from build123d import *

# Parameters (mm, degrees)
SKETCH1_R           = 1.75
SKETCH1_R_2         = 1.8
SKETCH1_R_3         = 1.7
BOSS_EXTRUDE1_DEPTH = 3


with BuildPart() as part:
    # Sketch1 → Boss-Extrude1 (new body)
    with BuildSketch(Plane.XY):
        with BuildLine():
            Line((-138, 334), (-123.000000001, 334))
            ThreePointArc((-123.000000001, 334), (-121.585786438, 333.414213562), (-121.000000001, 332))
            Line((-121.000000001, 332), (-121.000000001, 330))
            ThreePointArc((-121.000000001, 330), (-120.414213563, 328.585786438), (-119.000000001, 328))
            Line((-119.000000001, 328), (-79.825853915, 328))
            ThreePointArc((-79.825853915, 328), (-78.411640352, 327.414213562), (-77.825853915, 326))
            Line((-77.825853915, 326), (-77.825853915, 319))
            ThreePointArc((-77.825853915, 319), (-70.325853915, 311.5), (-62.825853915, 319))
            Line((-62.825853915, 319), (-62.825853915, 326))
            ThreePointArc((-62.825853915, 326), (-62.240067477, 327.414213562), (-60.825853915, 328))
            Line((-60.825853915, 328), (69.799384712, 328))
            ThreePointArc((69.799384712, 328), (71.213598275, 327.414213562), (71.799384712, 326))
            Line((71.799384712, 326), (71.799384712, 319))
            ThreePointArc((71.799384712, 319), (79.299384712, 311.5), (86.799384712, 319))
            Line((86.799384712, 319), (86.799384712, 326))
            ThreePointArc((86.799384712, 326), (87.38517115, 327.414213562), (88.799384712, 328))
            Line((88.799384712, 328), (119.000000001, 328))
            ThreePointArc((119.000000001, 328), (120.414213563, 328.585786438), (121.000000001, 330))
            Line((121.000000001, 330), (121.000000001, 332))
            ThreePointArc((121.000000001, 332), (121.585786438, 333.414213562), (123.000000001, 334))
            Line((123.000000001, 334), (138, 334))
            ThreePointArc((138, 334), (140.121320344, 333.121320344), (141, 331))
            Line((141, 331), (141, 227))
            ThreePointArc((141, 227), (140.121320344, 224.878679656), (138, 224))
            Line((138, 224), (-138, 224))
            ThreePointArc((-138, 224), (-140.121320344, 224.878679656), (-141, 227))
            Line((-141, 227), (-141, 331))
            ThreePointArc((-141, 331), (-140.121320344, 333.121320344), (-138, 334))
        make_face()
        with Locations((-131, 319)):
            Circle(SKETCH1_R, mode=Mode.SUBTRACT)
        with Locations((-131, 239)):
            Circle(SKETCH1_R, mode=Mode.SUBTRACT)
        with Locations((131, 319)):
            Circle(SKETCH1_R, mode=Mode.SUBTRACT)
        with Locations((131, 239)):
            Circle(SKETCH1_R, mode=Mode.SUBTRACT)
        with Locations((-104.5, 311.05)):
            Circle(SKETCH1_R, mode=Mode.SUBTRACT)
        with Locations((-94, 311.05)):
            Circle(SKETCH1_R, mode=Mode.SUBTRACT)
        with Locations((-103.8, 298.65)):
            Circle(SKETCH1_R, mode=Mode.SUBTRACT)
        with Locations((-85.9, 298.65)):
            Circle(SKETCH1_R, mode=Mode.SUBTRACT)
        with Locations((101.6, 312.25)):
            Circle(SKETCH1_R, mode=Mode.SUBTRACT)
        with Locations((112.2, 312.25)):
            Circle(SKETCH1_R, mode=Mode.SUBTRACT)
        with Locations((93.9, 298.55)):
            Circle(SKETCH1_R, mode=Mode.SUBTRACT)
        with Locations((112, 298.55)):
            Circle(SKETCH1_R, mode=Mode.SUBTRACT)
        with Locations((-50, 304)):
            Circle(SKETCH1_R, mode=Mode.SUBTRACT)
        with Locations((50, 304)):
            Circle(SKETCH1_R, mode=Mode.SUBTRACT)
        with Locations((8.910068617, 320.939971353)):
            Circle(SKETCH1_R_2, mode=Mode.SUBTRACT)
        with Locations((48.910068617, 320.939971353)):
            Circle(SKETCH1_R_2, mode=Mode.SUBTRACT)
        with Locations((-113.4, 285.5)):
            Circle(SKETCH1_R_3, mode=Mode.SUBTRACT)
        with Locations((-16.54, 280.5)):
            Circle(SKETCH1_R, mode=Mode.SUBTRACT)
        with Locations((-5.5, 280.5)):
            Circle(SKETCH1_R, mode=Mode.SUBTRACT)
        with Locations((13.46, 280.5)):
            Circle(SKETCH1_R, mode=Mode.SUBTRACT)
        with Locations((-113.4, 249.2)):
            Circle(SKETCH1_R_3, mode=Mode.SUBTRACT)
        with Locations((-61.5, 249.2)):
            Circle(SKETCH1_R_3, mode=Mode.SUBTRACT)
        with Locations((-61.5, 292.2)):
            Circle(SKETCH1_R_3, mode=Mode.SUBTRACT)
        with Locations((24.5, 280.5)):
            Circle(SKETCH1_R, mode=Mode.SUBTRACT)
        with Locations((43.46, 280.5)):
            Circle(SKETCH1_R, mode=Mode.SUBTRACT)
        with Locations((54.5, 280.5)):
            Circle(SKETCH1_R, mode=Mode.SUBTRACT)
        with Locations((-20.870942191, 310.54)):
            Circle(SKETCH1_R, mode=Mode.SUBTRACT)
        with Locations((-20.870942191, 299.5)):
            Circle(SKETCH1_R, mode=Mode.SUBTRACT)
        with Locations((78.5, 290.5)):
            Circle(SKETCH1_R, mode=Mode.SUBTRACT)
        with Locations((78.5, 279.46)):
            Circle(SKETCH1_R, mode=Mode.SUBTRACT)
    extrude(amount=BOSS_EXTRUDE1_DEPTH)


solid = part.part
The model under review builds one solid part; all positions refer to its coordinate system, in mm. Give positions to 0.01 mm unless a question says otherwise; leave off trailing zeros. Write each loop counter-clockwise with the first axis right and the second up, starting at its lowest first coordinate (ties: lowest second). Pieces come first, ordered by that corner, then holes.
1. Add section B-B, the plane z = 2.3. Count the separate pieces of the cut face and the enclosed holes in it, plus the area to 3 significant figures.
2. For P1, Ø4.5, axis at x = 24.5, y = 280.5, coming from the +Z side; P2, Ø1.5, axis at x = -106, z = 1.5, coming from the +Y side, all flat-tipped, find the tip position at first contact; note any pin that passes through.
3. Wall thickness on L1, parallel to Y at x = 78.5, z = 1; L2, parallel to Y at x = -113.4, z = 2.05; L3, parallel to X at y = 304, z = 1: over which ranges is each line inside the solid? List them lowest first.
4. Add section C-C, the plane x = -71. Write out the cut boundary in (y, z), plus the area to 3 significant figures.
5. Add section A-A, the plane x = -33.5. Write out the cut boundary in (y, z).
Worked answers:
1. separate pieces: 1
1. enclosed holes: 30
1. area: 28,800 mm2
2. P1: stops at z = 3
2. P2: stops at y = 328
3. L1: y = 224 to 277.71, 281.21 to 288.75, 292.25 to 311.54
3. L2: y = 224 to 247.5, 250.9 to 283.8, 287.2 to 328
3. L3: x = -141 to -51.75, -48.25 to 48.25, 51.75 to 141
4. outline: (224, 0) - (311.53, 0) - (311.53, 3) - (224, 3) - close
4. area: 263 mm2
5. outline: (224, 0) - (328, 0) - (328, 3) - (224, 3) - close
